Geometry: see drawing. Coordinates: mm, zero at the bounding-box minimum. Round coordinates to 2 decimals unless told otherwise and drop trailing zeros. Order: outer loops, then holes, each group sorted by start corner. A loop starts at its lowest first (then second) coordinate and runs counter-clockwise, first axis right, second up. Notation, with made-up numbers: (57, 71) -> (74, 71) arc R32 cw to (74, 110) -> close; hole circle Ø9 at (39.25, 22). An arc over 180 degrees is marked (long way). Put each result on its own line as item: value.
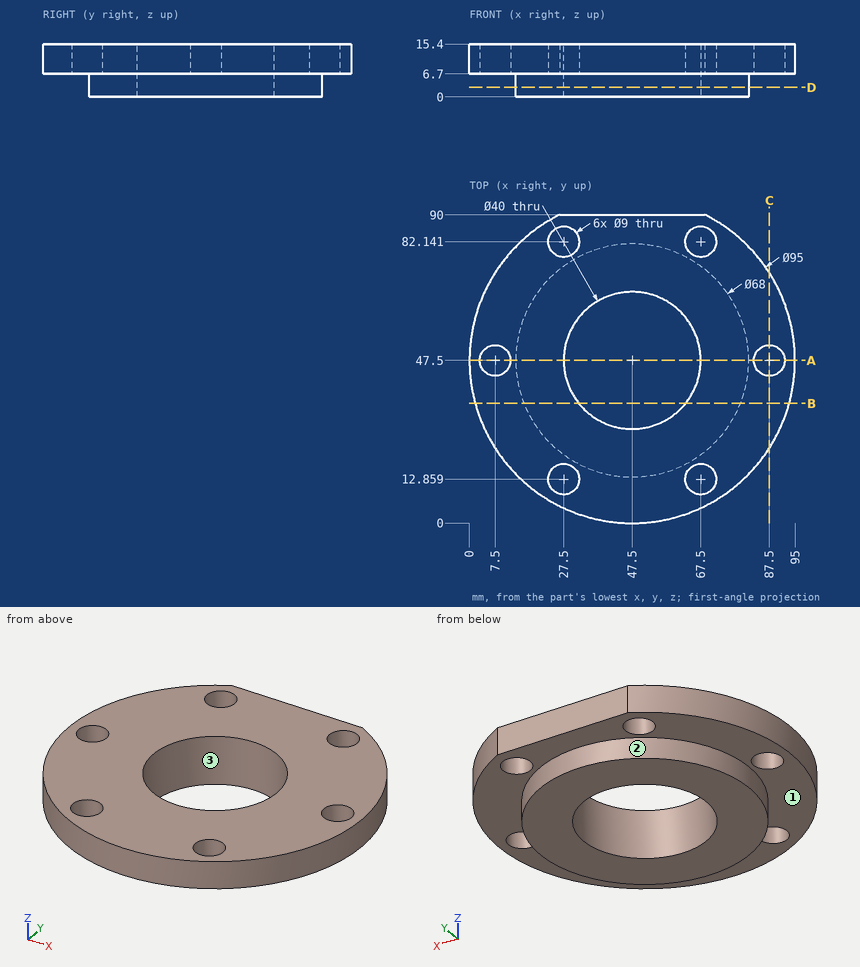
1. Cut plane D-D on z = 2.75. Return loops of the section in (x, y).
Ans:
outline: circle Ø68 at (47.5, 47.5); hole circle Ø40 at (47.5, 47.5)
2. Draft query along X for the marked faces 1, 2 and 3. Return one class per face: +X half, -X half, draft (parallel to the pull), parting line (faces both ways), or undercut.
Ans:
face 1: draft
face 2: parting line
face 3: undercut
3. Contact query for flat-ended pins moving along their axis: P1, Ø5, axis at y = 55.5, z = 9, coming from the +X side; P2, Ø5, axis at y = 74, z = 4, coming from the -X side; P3, Ø5.5, axis at x = 67.5, y = 82.14, coming from the -Z side; P4, Ø6, axis at x = 13, y = 28, coming from the -Z side. Output: stop coordinate, or through.
Ans:
P1: x = 94.68
P2: x = 23.42
P3: through
P4: z = 6.7
4. Cut plane A-A on y = 47.5. Return loops of the section in (x, z), and give its area (4 significant figures).
Ans:
outline: (0, 6.7) -> (3, 6.7) -> (3, 15.4) -> (0, 15.4) -> close; (12, 6.7) -> (13.5, 6.7) -> (13.5, 0) -> (27.5, 0) -> (27.5, 15.4) -> (12, 15.4) -> close; (67.5, 0) -> (81.5, 0) -> (81.5, 6.7) -> (83, 6.7) -> (83, 15.4) -> (67.5, 15.4) -> close; (92, 6.7) -> (95, 6.7) -> (95, 15.4) -> (92, 15.4) -> close
area: 509.5 mm²
5. Cut plane B-B on y = 35. Return loops of the section in (x, z), and give its area (3 significant figures).
Ans:
outline: (1.67, 6.7) -> (15.88, 6.7) -> (15.88, 0) -> (31.89, 0) -> (31.89, 15.4) -> (1.67, 15.4) -> close; (63.11, 0) -> (79.12, 0) -> (79.12, 6.7) -> (93.33, 6.7) -> (93.33, 15.4) -> (63.11, 15.4) -> close
area: 740 mm²
6. Cut plane C-C on x = 87.5. Return loops of the section in (y, z), and give its area (3 significant figures).
Ans:
outline: (21.88, 6.7) -> (43, 6.7) -> (43, 15.4) -> (21.88, 15.4) -> close; (52, 6.7) -> (73.12, 6.7) -> (73.12, 15.4) -> (52, 15.4) -> close
area: 367 mm²
7. Material intervals for probe 1 along Y at (x, z) = (65.5, 9.75); probe 2 along X at (y, z) = (48.5, 9.5) (1 decimal); probe 3 along Z at (x, y) = (17, 30), sorted ascending.
Ans:
probe 1: 3.54 to 8.83, 16.89 to 38.78, 56.22 to 78.11, 86.17 to 90
probe 2: 0 to 3.1, 11.9 to 27.5, 67.5 to 83.1, 91.9 to 95
probe 3: 6.7 to 15.4
